Source: CAD feature listing. Evaluate the final solid. Frame: model axes, mm. Give positions to 0.01 mm unless a question says otherwise; leave off trailing zeros. Order: outer loops, then holes, each group sorted by start corner. A loop starts at its lowest first (then second) coordinate and runs counter-clockwise, first axis right, second up. Notation, with made-up numbers: (71, -36) - (130, -36) arc R22 cw to (130, -1) - close; hole circle Ø5 at (12.5, 1). An arc over 180 degrees is marked (long way). Write each question's results on one line, items separated by ' | '. Start each with the question number.
Item 1: Line query: line 1 along X through (y, z) = (3.75, -76.2); line 2 along Z through (x, y) = (0, 1.75). Output: solid intervals per line, ascending.
Item 2: Section A-A on x = 0. Output: boundary loops of the cut face in (y, z).
Item 3: Mould query, pull axis Z, two halves, no side actions, for faces 1 (the flat face through (-1, 6.35, -1)), 2 (the flat face through (-1, 3, -82.55)), 3 (the cylindrical face through (-73.65, 3.13, -0.11)). Classes: released by +Z, released by -Z, zero draft, split by the parting line, or undercut.
```python
from build123d import *

# Parameters (mm, degrees)
SKETCH1_W              = 165.1
SKETCH1_H              = 165.1
BOSS_EXTRUDE1_DEPTH    = 6.35
FILLET1_R              = 6.35
F_10_CLEARANCE_HOLE1_D = 5.1054


with BuildPart() as part:
    # Sketch1 → Boss-Extrude1 (new body)
    with BuildSketch(Plane(origin=(0, 0, 0), x_dir=(1, 0, 0), z_dir=(0, 1, 0))):
        Rectangle(SKETCH1_W, SKETCH1_H)
    extrude(amount=BOSS_EXTRUDE1_DEPTH)

    # Fillet1
    fillet1_edges = [part.edges().sort_by_distance(p)[0] for p in [
        (-82.55, 3.175, -82.55),
        (82.55, 3.175, -82.55),
        (82.55, 3.175, 82.55),
        (-82.55, 3.175, 82.55),
    ]]
    fillet(fillet1_edges, radius=FILLET1_R)

    # #10 Clearance Hole1 (through all)
    with Locations(Plane(origin=(0, 6.35, 0), x_dir=(1, 0, 0), z_dir=(0, 1, 0))):
        with Locations((-76.2, -76.2), (-76.2, 76.2), (76.2, 76.2), (76.2, -76.2), (0, 76.2), (0, -76.2), (-76.2, 0), (76.2, 0)):
            Hole(F_10_CLEARANCE_HOLE1_D / 2)


solid = part.part
```
Evaluation:
1) line 1: x = -82.55 to -78.75, -73.65 to -2.55, 2.55 to 73.65, 78.75 to 82.55 | line 2: z = -82.55 to -78.75, -73.65 to 73.65, 78.75 to 82.55
2) outline: (0, -82.55) - (6.35, -82.55) - (6.35, -78.75) - (0, -78.75) - close; (0, -73.65) - (6.35, -73.65) - (6.35, 73.65) - (0, 73.65) - close; (0, 78.75) - (6.35, 78.75) - (6.35, 82.55) - (0, 82.55) - close
3) face 1: zero draft | face 2: released by -Z | face 3: undercut
